CAD build for the part. Positions are in the model's coordinates, mm. Give positions to 0.01 mm unless a question says otherwise; leave off trailing zeros. Order: outer loops, then holes, each group sorted by start corner. A loop starts at its lowest first (then second) coordinate and runs counter-clockwise, first axis right, second up.
from build123d import *

# Parameters (mm, degrees)
SKETCH1_R             = 47.5
SKETCH1_R_2           = 21.55
BOSS_EXTRUDE1_DEPTH   = 1.5
F_3_0MM_DOWEL_HOLE1_D = 3
CIRPATTERN1_COUNT     = 9
BOSS_EXTRUDE2_DEPTH   = 1.5
FILLET7_R             = 10
FILLET8_R             = 10
FILLET9_R             = 1
FILLET10_R            = 1
CUT_EXTRUDE2_DEPTH    = 1.5


with BuildPart() as part:
    # Sketch1 → Boss-Extrude1 (new body)
    with BuildSketch(Plane.XY):
        Circle(SKETCH1_R)
        Circle(SKETCH1_R_2, mode=Mode.SUBTRACT)
    extrude(amount=BOSS_EXTRUDE1_DEPTH)

    # Ø3.0mm Dowel Hole1 (through all)
    with Locations(Plane.XY.offset(1.5)):
        with Locations((0, 36.5)):
            f_3_0mm_dowel_hole1 = Hole(F_3_0MM_DOWEL_HOLE1_D / 2)

    # CirPattern1: Ø3.0mm Dowel Hole1 ×9 about axis
    cirpattern1_axis = Axis((0, 0, 0), (0, 0, 1))
    for i in range(1, CIRPATTERN1_COUNT):
        add(f_3_0mm_dowel_hole1.rotate(cirpattern1_axis, i * 360 / CIRPATTERN1_COUNT), mode=Mode.SUBTRACT)

    # Sketch6 → Boss-Extrude2 (add)
    with BuildSketch(Plane.XY.offset(1.5)):
        Polygon((-25.563438214, -40.034492962), (25.563438214, -40.034492962), (25.563438214, -166.774492962), (30.563438214, -166.774492962), (30.563438214, -196.784492962), (25.563438214, -201.784492962), (-25.563438214, -202.2867607), (-30.563438214, -196.784492962), (-30.563438214, -166.784492962), (-25.563438214, -166.784492962), align=None)
    extrude(amount=-BOSS_EXTRUDE2_DEPTH)

    # Fillet7
    fillet7_edges = [part.edges().sort_by_distance(p)[0] for p in [
        (-25.563438214, -40.034492962, 0.75),
    ]]
    fillet(fillet7_edges, radius=FILLET7_R)

    # Fillet8
    fillet8_edges = [part.edges().sort_by_distance(p)[0] for p in [
        (25.563438214, -40.034492962, 0.75),
    ]]
    fillet(fillet8_edges, radius=FILLET8_R)

    # Fillet9
    fillet9_edges = [part.edges().sort_by_distance(p)[0] for p in [
        (30.563438214, -166.774492962, 0.75),
        (-30.563438214, -166.784492962, 0.75),
    ]]
    fillet(fillet9_edges, radius=FILLET9_R)

    # Fillet10
    fillet10_edges = [part.edges().sort_by_distance(p)[0] for p in [
        (30.563438214, -196.784492962, 0.75),
        (25.563438214, -201.784492962, 0.75),
        (-25.563438214, -202.2867607, 0.75),
        (-30.563438214, -196.784492962, 0.75),
    ]]
    fillet(fillet10_edges, radius=FILLET10_R)

    # Sketch8 → Cut-Extrude2 (cut)
    with BuildSketch(Plane(origin=(0, 0, 0), x_dir=(-1, 0, 0), z_dir=(0, 0, -1))):
        with BuildLine():
            Line((-7.519953185, -145.285430812), (-7.519953185, -119.885430812))
            ThreePointArc((-7.519953185, -119.885430812), (-0.019953185, -112.385430812), (7.480046815, -119.885430812))
            Line((7.480046815, -119.885430812), (7.480046815, -145.285430812))
            ThreePointArc((7.480046815, -145.285430812), (-0.019953185, -152.785430812), (-7.519953185, -145.285430812))
        make_face()
    extrude(amount=-CUT_EXTRUDE2_DEPTH, mode=Mode.SUBTRACT)


solid = part.part
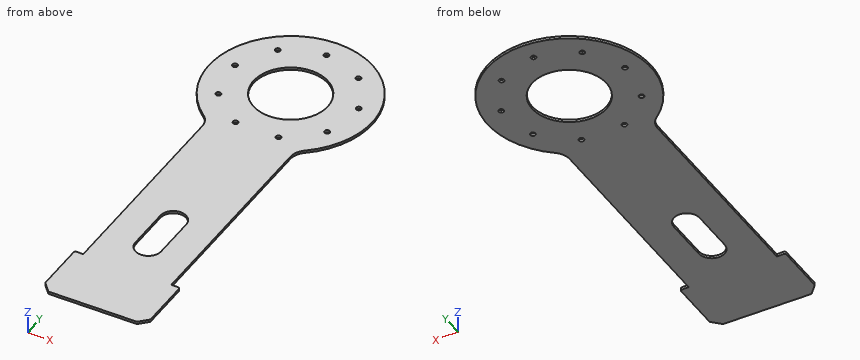
1. Wall check: line 1 (X direction, y = 5.5, z = 0.7); line 2 (X direction, y = -162.5, z = 1.2); line 3 (Y direction, x = -35, z = 0.3). Give the ranges that are in metal, low to high.
2. Saw through at C-C on x = 17. Give the cut face in (y, z), plus the area to 3 significant figures.
3. Saw through at A-A on y = 0. Give the cut face in (x, z), plus the area to 4 significant figures.
4. Saw through at D-D on y = -155. Give the cut face in (x, z), plus the area to 3 significant figures.
5. Pin check, flat tips, straight feed: P1, Ø0.8, axis at y = -127, z = 1, coming from the -X side; P2, Ø0.8, axis at x = -27, z = 1, coming from the +Y side; P3, Ø0.8, axis at x = 28, z = 1, coming from the +Y side. Stop position of each tip, or through.
6. Saw through at B-B on z = 1.2. State how many separate pieces and enclosed holes the cut face has, plus the area to 3 significant figures.
Reported:
1. line 1: x = -47.18 to -37.19, -34.7 to -20.84, 20.84 to 34.7, 37.19 to 47.18
1. line 2: x = -25.56 to 25.56
1. line 3: y = -32.11 to 5.17, 7.5 to 32.11
2. outline: (-201.87, 0) - (-13.24, 0) - (-13.24, 1.5) - (-201.87, 1.5) - close; (13.24, 0) - (44.35, 0) - (44.35, 1.5) - (13.24, 1.5) - close
2. area: 330 mm2
3. outline: (-47.5, 0) - (-21.55, 0) - (-21.55, 1.5) - (-47.5, 1.5) - close; (21.55, 0) - (47.5, 0) - (47.5, 1.5) - (21.55, 1.5) - close
3. area: 77.85 mm2
4. outline: (-25.56, 0) - (25.56, 0) - (25.56, 1.5) - (-25.56, 1.5) - close
4. area: 76.7 mm2
5. P1: stops at x = -25.56
5. P2: stops at y = 39.35
5. P3: stops at y = 38.66
6. separate pieces: 1
6. enclosed holes: 11
6. area: 13,400 mm2
